For this review, take the finished solid that the model builds, in its own axes (mm). Give positions to 0.01 mm unless a question says otherwise; leave off trailing zeros. Write each loop counter-clockwise with the first axis right and the second up, starting at its lowest first coordinate (ties: lowest second). Pieces come first, ordered by that corner, then holes. Notation, with made-up numbers: M 45.25,73 L 89.25,73 A24 cw 89.25,99 Z; hole C -10.5,82 d8. An arc over 180 degrees is marked long. One line per item, written item: value. Start each with the question number.
Item 1: Consider section B-B, the plane z = -73. Write out the cut boundary in (x, y).
Item 2: To check wall thickness, follow probe 1 along X at (y, z) = (4.25, -137); probe 2 along Y at (x, z) = (-9.75, -173.2). State the ranges of each line that lie inside material, in increasing order.
Item 3: Consider section A-A, the plane y = -6.5. Write out the cut boundary in (x, z), and give its area (3 significant figures).
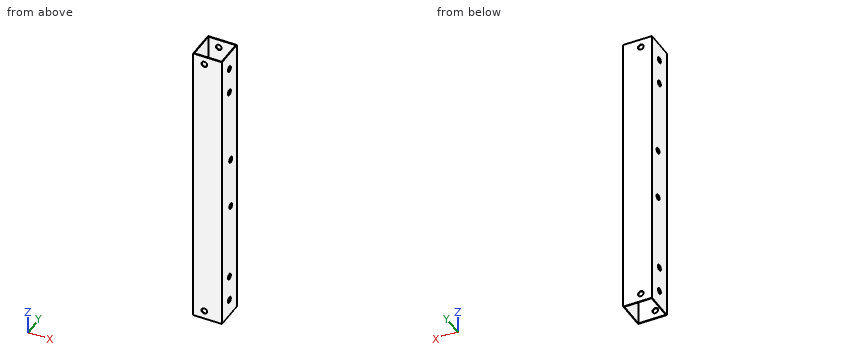
```python
from build123d import *

# Parameters (mm, degrees)
SKETCH_1_W          = 20
SKETCH_1_H          = 20
SKETCH_1_W_2        = 19
SKETCH_1_H_2        = 19
EXTRUDE_1_DEPTH     = 203.2
SKETCH_2_R          = 2
CUT_EXTRUDE_1_DEPTH = 205.426612749
SKETCH_3_R          = 2
CUT_EXTRUDE_2_DEPTH = 205.426612749


with BuildPart() as part:
    # 草图1 → 凸台-拉伸1 (new body)
    with BuildSketch(Plane.XY):
        Rectangle(SKETCH_1_W, SKETCH_1_H)
        Rectangle(SKETCH_1_W_2, SKETCH_1_H_2, mode=Mode.SUBTRACT)
    extrude(amount=-EXTRUDE_1_DEPTH)

    # 草图2 → 切除-拉伸1 (cut, through all)
    with BuildSketch(Plane.ZY.offset(10)):
        with Locations(Location((-30, 0, 0), (0, 0, 270))):
            Circle(SKETCH_2_R)
        with Locations(Location((-83.6, 1.794910396, 0), (0, 0, 270))):
            Circle(SKETCH_2_R)
        with Locations(Location((-119.6, 1.794910396, 0), (0, 0, 270))):
            Circle(SKETCH_2_R)
        with Locations(Location((-173.2, 0, 0), (0, 0, 270))):
            Circle(SKETCH_2_R)
        with Locations(Location((-191.2, 0, 0), (0, 0, 270))):
            Circle(SKETCH_2_R)
        with Locations(Location((-12, 0, 0), (0, 0, 270))):
            Circle(SKETCH_2_R)
    extrude(amount=-CUT_EXTRUDE_1_DEPTH, mode=Mode.SUBTRACT)

    # 草图3 → 切除-拉伸2 (cut, through all)
    with BuildSketch(Plane(origin=(0, 10, 0), x_dir=(1, 0, 0), z_dir=(0, 1, 0))):
        with Locations(Location((-2.25, 197.371407716, 0), (0, 0, 270))):
            Circle(SKETCH_3_R)
        with Locations(Location((-2.25, 5.828592284, 0), (0, 0, 270))):
            Circle(SKETCH_3_R)
    extrude(amount=-CUT_EXTRUDE_2_DEPTH, mode=Mode.SUBTRACT)


solid = part.part
```
Model answer:
1. outline: M -10,-10 L 10,-10 L 10,10 L -10,10 Z; hole M -9.5,-9.5 L 9.5,-9.5 L 9.5,9.5 L -9.5,9.5 Z
2. probe 1: x = -10 to -9.5, 9.5 to 10
2. probe 2: y = -10 to -2, 2 to 10
3. outline: M -10,-203.2 L -9.5,-203.2 L -9.5,0 L -10,0 Z; M 9.5,-203.2 L 10,-203.2 L 10,0 L 9.5,0 Z
3. area: 203 mm2
